Study the drawing (mm; zero at the part's minimum x, y, z) and answer. A direction names the side the tool comes from. Coordinates: 2 decimals unless noted, no trailing zeros. Loops run counter-clockwise (first coordinate to the right, second up) from the corner with the lowest first, then second, coordinate; pieces in that order, holes last.
Q1. Section B-B (x = 17) is taken. Give the vertices of the cut face in (y, z), then the cut area to 3 significant figures.
Q2. Flat-ended cylindrical pins translate along their axes: P1, Ø3.5, axis at x = 28.5, y = 15, coming from the -Z side; P2, Ø10, axis at x = 63.5, y = 4, coming from the +Z side; P3, Ø1.2, axis at x = 37, z = 3.5, coming from the +Y side (1 decimal). Find the tip coordinate at first contact, or state that the pin passes through.
Q3. Section D-D (z = 27.5) is taken. Give the vertices of the cut face in (x, y) (1 decimal).
Q4. Section C-C (y = 6) is taken. Give the vertices of the cut face in (x, z).
Q5. The mould has two halves that part along X. Classify the marked faces 6, 7, 8 and 9: pulls with the +X half, pulls with the -X half, needs draft (parallel to the pull), parting line crosses it, or undercut.
Q6. Section A-A (y = 16) is taken. Give the vertices of the cut face in (x, z).
Q7. Straight lines are drawn through the part: line 1 (X direction, y = 20, z = 12) (1 decimal); line 2 (X direction, y = 30.5, z = 14); line 3 (Y direction, x = 37, z = 13) (1 decimal). For each, find the intervals that lie inside material, in ascending order.
Q8. Which of the six approach directions +Z, -Z, +X, -X, +Y, -Y give full straight-line access (tool end or side, diameter ignored) to the marked faces 1, 2, 3, 4 and 5?
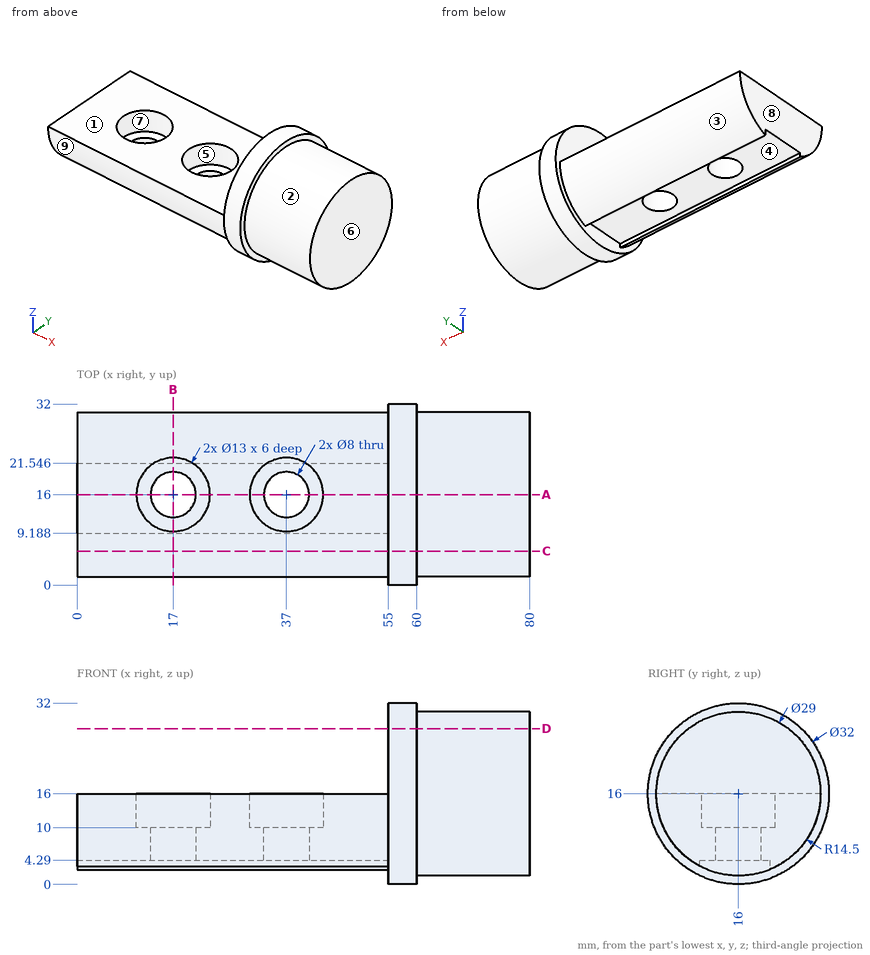
Numbers:
1. outline: (1.5, 16) arc R14.5 ccw to (9.19, 3.2) - (9.19, 4.29) - (12, 4.29) - (12, 10) - (9.5, 10) - (9.5, 16) - close; (20, 4.29) - (21.55, 4.29) - (21.55, 2.6) arc R14.5 ccw to (30.5, 16) - (22.5, 16) - (22.5, 10) - (20, 10) - close
1. area: 178 mm2
2. P1: stops at z = 4.29
2. P2: stops at z = 29.6
2. P3: stops at y = 24.3
3. outline: (55, 4.9) - (60, 4.9) - (60, 7.2) - (80, 7.2) - (80, 24.8) - (60, 24.8) - (60, 27.1) - (55, 27.1) - close
4. outline: (0, 5.5) - (55, 5.5) - (55, 3.51) - (60, 3.51) - (60, 5.5) - (80, 5.5) - (80, 26.5) - (60, 26.5) - (60, 28.49) - (55, 28.49) - (55, 16) - (0, 16) - close
5. face 6: pulls with the +X half
5. face 7: undercut
5. face 8: pulls with the -X half
5. face 9: needs draft
6. outline: (0, 4.29) - (13, 4.29) - (13, 10) - (10.5, 10) - (10.5, 16) - (0, 16) - close; (21, 4.29) - (33, 4.29) - (33, 10) - (30.5, 10) - (30.5, 16) - (23.5, 16) - (23.5, 10) - (21, 10) - close; (41, 4.29) - (55, 4.29) - (55, 0) - (60, 0) - (60, 1.5) - (80, 1.5) - (80, 30.5) - (60, 30.5) - (60, 32) - (55, 32) - (55, 16) - (43.5, 16) - (43.5, 10) - (41, 10) - close
7. line 1: x = 0 to 11.9, 22.1 to 31.9, 42.1 to 80
7. line 2: x = 55 to 60
7. line 3: y = 1.8 to 9.5, 22.5 to 30.2
8. face 1: +Z, -X, +Y, -Y
8. face 2: +X
8. face 3: -Z, -X, +Y
8. face 4: -Z, -X
8. face 5: +Z
